Here's how the part is built. I have some questions about the finished solid (model axes, mm). Face numbers are marked on the shaded views. A direction names the side the tool comes from. Round coordinates to 2 decimals unless told otherwise and drop trailing zeros. Order: outer loops, then holes, each group sorted by start corner. A loop starts at its lowest first (then second) coordinate and runs counter-clockwise, first axis right, second up.
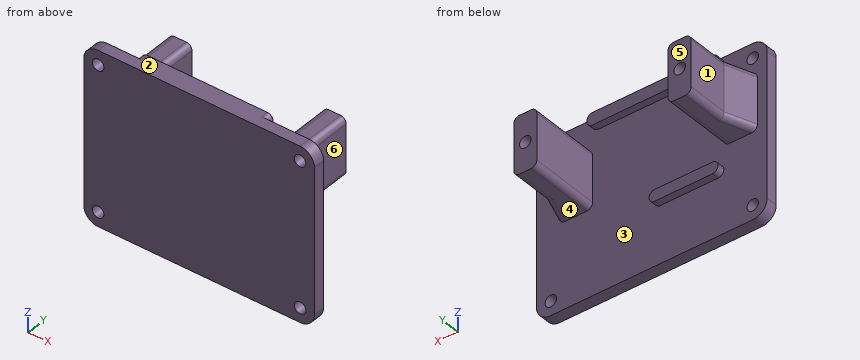
```python
from build123d import *
from OCP.BRepFilletAPI import BRepFilletAPI_MakeChamfer

# Parameters (mm, degrees)
SKETCH_1_W          = 80
SKETCH_1_H          = 60
SKETCH_1_R          = 2
EXTRUDE_1_DEPTH     = 4
FILLET_1_R          = 5
SKETCH_2_W          = 24
SKETCH_2_H          = 4
SKETCH_2_W_2        = 45.5
SKETCH_2_H_2        = 4.25
EXTRUDE_2_DEPTH     = 2.5
EXTRUDE_3_DEPTH     = 24.5
SKETCH_3_R          = 2
CUT_EXTRUDE_1_DEPTH = 7
CHAMFER_1_SIZE      = 10
CHAMFER_1_SIZE2     = 3.639702343
FILLET_2_R          = 2
FILLET_3_R          = 2
FILLET_4_R          = 2


with BuildPart() as part:
    # Эскиз1 → Бобышка-Вытянуть1 (new body)
    with BuildSketch(Plane(origin=(0, 0, 0), x_dir=(1, 0, 0), z_dir=(0, 1, 0))):
        Rectangle(SKETCH_1_W, SKETCH_1_H)
        with Locations(Location((-35, 25, 0), (0, 0, 270))):
            Circle(SKETCH_1_R, mode=Mode.SUBTRACT)
        with Locations(Location((35, 25, 0), (0, 0, 270))):
            Circle(SKETCH_1_R, mode=Mode.SUBTRACT)
        with Locations(Location((-35, -25, 0), (0, 0, 270))):
            Circle(SKETCH_1_R, mode=Mode.SUBTRACT)
        with Locations(Location((35, -25, 0), (0, 0, 270))):
            Circle(SKETCH_1_R, mode=Mode.SUBTRACT)
    extrude(amount=EXTRUDE_1_DEPTH)

    # Скругление1
    fillet_1_edges = [part.edges().sort_by_distance(p)[0] for p in [
        (40, 2, 30),
        (-40, 2, 30),
        (-40, 2, -30),
        (40, 2, -30),
    ]]
    fillet(fillet_1_edges, radius=FILLET_1_R)

    # Эскиз2 → Бобышка-Вытянуть2 (add)
    with BuildSketch(Plane(origin=(0, 4, 0), x_dir=(1, 0, 0), z_dir=(0, 1, 0))):
        with Locations((-13, 8.25)):
            Rectangle(SKETCH_2_W, SKETCH_2_H)
        with Locations((-2.25, -27.875)):
            Rectangle(SKETCH_2_W_2, SKETCH_2_H_2)
    extrude(amount=EXTRUDE_2_DEPTH)

    # Эскиз2<3> → Бобышка-Вытянуть3 (add)
    with BuildSketch(Plane(origin=(0, 4, 0), x_dir=(1, 0, 0), z_dir=(0, 1, 0))):
        Polygon((20.5, -19.75), (20.5, -9.75), (20.5, 0.25), (28.5, 0.25), (28.5, -19.75), align=None)
        Polygon((-25, -19.75), (-25, -9.75), (-25, 0.25), (-33, 0.25), (-33, -19.75), align=None)
    extrude(amount=EXTRUDE_3_DEPTH)

    # Эскиз3 → Вырез-Вытянуть1 (cut)
    with BuildSketch(Plane(origin=(0, 28.5, 0), x_dir=(1, 0, 0), z_dir=(0, 1, 0))):
        with Locations(Location((-29, -9.75, 0), (0, 0, 270))):
            Circle(SKETCH_3_R)
        with Locations(Location((24.5, -9.75, 0), (0, 0, 270))):
            Circle(SKETCH_3_R)
    extrude(amount=-CUT_EXTRUDE_1_DEPTH, mode=Mode.SUBTRACT)

    # Фаска1: one chamfer whose edges measure the first distance from different faces: ONE call of the kernel's chamfer builder (chamfer() names one face for all edges)
    chamfer_1_edges_1 = [part.edges().sort_by_distance(p)[0] for p in [
        (28.5, 4, 9.75),
    ]]
    chamfer_1_side_1 = [part.faces().sort_by_distance(p)[0] for p in [
        (28.5, 16.25, 9.75),
    ]]
    chamfer_1_edges_2 = [part.edges().sort_by_distance(p)[0] for p in [
        (-33, 4, 9.75),
    ]]
    chamfer_1_side_2 = [part.faces().sort_by_distance(p)[0] for p in [
        (-33, 16.25, 9.75),
    ]]
    chamfer_1 = BRepFilletAPI_MakeChamfer(part.part.solid().wrapped)
    for e in chamfer_1_edges_1:
        chamfer_1.Add(CHAMFER_1_SIZE, CHAMFER_1_SIZE2, e.wrapped, chamfer_1_side_1[0].wrapped)  # the first distance lies on this face
    for e in chamfer_1_edges_2:
        chamfer_1.Add(CHAMFER_1_SIZE, CHAMFER_1_SIZE2, e.wrapped, chamfer_1_side_2[0].wrapped)  # the first distance lies on this face
    add(Compound.cast(chamfer_1.Shape()), mode=Mode.REPLACE)

    # Скругление2
    fillet_2_edges = [part.edges().sort_by_distance(p)[0] for p in [
        (-34.819851171, 9, 19.75),
        (-34.819851171, 9, -0.25),
        (30.319851171, 9, 19.75),
        (30.319851171, 9, -0.25),
        (20.5, 16.25, -0.25),
        (20.5, 16.25, 19.75),
        (-25, 16.25, 19.75),
        (-25, 16.25, -0.25),
    ]]
    fillet(fillet_2_edges, radius=FILLET_2_R)

    # Скругление3
    fillet_3_edges = [part.edges().sort_by_distance(p)[0] for p in [
        (-25, 5.25, -6.25),
        (-1, 5.25, -10.25),
        (-25, 5.25, -10.25),
        (-1, 5.25, -6.25),
        (20.5, 5.25, 25.75),
        (20.5, 5.25, 30),
        (-25, 5.25, 30),
        (-25, 5.25, 25.75),
    ]]
    fillet(fillet_3_edges, radius=FILLET_3_R - 0.0001)  # a hair under: the kernel refuses the full size

    # Скругление4
    fillet_4_edges = [part.edges().sort_by_distance(p)[0] for p in [
        (28.5, 18.3261956, -0.25),
        (28.5, 18.3261956, 19.75),
        (-33, 18.3261956, -0.25),
        (-33, 18.3261956, 19.75),
    ]]
    fillet(fillet_4_edges, radius=FILLET_4_R)


solid = part.part
```
1. If we section it at C-C, the plane x = -29: Write out the boundary of the cut face in (y, z).
Evaluation:
outline: (0, -30) - (4, -30) - (4, -0.25) - (28.5, -0.25) - (28.5, 7.75) - (21.5, 7.75) - (21.5, 11.75) - (28.5, 11.75) - (28.5, 19.75) - (4, 19.75) - (4, 30) - (0, 30) - close
2. I'm going to push flat-ended pins straight in: P1, Ø3, axis at y = 4.5, z = 16, coming from the -X side; P2, Ø5, axis at y = 7, z = 1, coming from the +X side; P3, Ø8.5, axis at x = 27, y = 19.5, coming from the +Z side; P4, Ø11.5, axis at y = 18, z = 11.5, coming from the +X side. Where does each tip first touch, or does it pass through?
Evaluation:
P1: stops at x = -40
P2: stops at x = 31.93
P3: stops at z = 19.75
P4: stops at x = 29.14
3. If we mould it in two halves opening along X, with no side actions, what happens to the marked faces 1, 2 and 3? For each: released by +X, released by -X, zero draft, split by the parting line, or undercut.
Evaluation:
face 1: released by -X
face 2: zero draft
face 3: undercut
4. On a 3-axis mill with a long thin cutter (end or side, diameter ignored), from which of +Z, -Z, +X, -X, +Y, -Y can I reach the whole of each face in a straight line? I mean the marked faces 4, 5 and 6. Say none if no direction works.
Evaluation:
face 4: -Z, +X, -X, +Y
face 5: +Z, -Z, +X, -X, +Y
face 6: +Z, -Z, +X, +Y
5. If we section it at B-B, the plane z = 9.75: Write out the boundary of the cut face in (x, y).
Evaluation:
outline: (-40, 0) - (40, 0) - (40, 4) - (32.14, 4) - (28.5, 14) - (28.5, 28.5) - (26.5, 28.5) - (26.5, 21.5) - (22.5, 21.5) - (22.5, 28.5) - (20.5, 28.5) - (20.5, 4) - (-25, 4) - (-25, 28.5) - (-27, 28.5) - (-27, 21.5) - (-31, 21.5) - (-31, 28.5) - (-33, 28.5) - (-33, 14) - (-36.64, 4) - (-40, 4) - close
6. If we section it at D-D, the plane z = 21.5: Write out the boundary of the cut face in (x, y).
Evaluation:
outline: (-40, 0) - (40, 0) - (40, 4) - (-40, 4) - close
7. I need wall thicknesses on probe 1 along X at (y, z) = (2.4, -25); probe 2 along X at (y, z) = (25, 9.75); probe 3 along X at (y, z) = (21.5, 7.5). Which ranges of each line are inside material? Lowest first, please.
Evaluation:
probe 1: x = -40 to -37, -33 to 33, 37 to 40
probe 2: x = -33 to -31, -27 to -25, 20.5 to 22.5, 26.5 to 28.5
probe 3: x = -33 to -25, 20.5 to 28.5
8. If we section it at A-A, the plane x = 0.5: Write out the boundary of the cut face in (y, z), and give its area (3 significant figures).
Evaluation:
outline: (0, -30) - (4, -30) - (4, 25.75) - (6.5, 25.75) - (6.5, 30) - (0, 30) - close
area: 251 mm2
